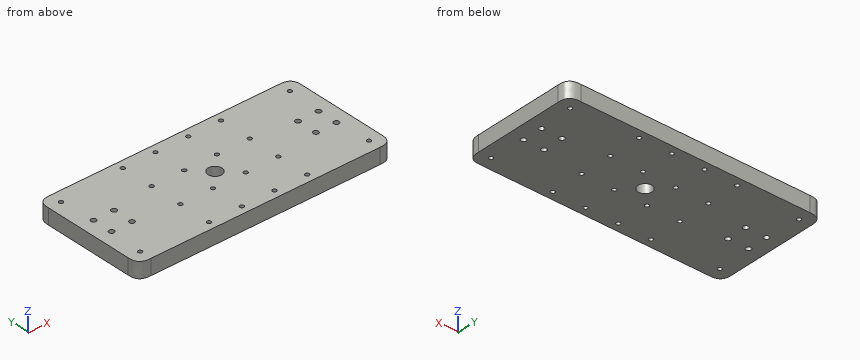
from build123d import *

# Parameters (mm, degrees)
SKETCH1_W                           = 310
SKETCH1_H                           = 140
BOSS_EXTRUDE1_DEPTH                 = 19.05
TAP_DRILL_FOR_M6X1_0_TAP1_D         = 5
LPATTERN1_COUNT                     = 4
LPATTERN1_PITCH                     = 40
LPATTERN1_COUNT_DIR2                = 4
LPATTERN1_PITCH_DIR2                = 40
FILLET1_SIZE                        = 15
M6_CLEARANCE_HOLE1_D                = 6.4
M16_CLEARANCE_HOLE1_D               = 17
TAP_START                           = -1
TAP_DRILL_FOR_M6X1_0_TAP2_OUTLINE_R = 2.5
TAP_DRILL_FOR_M6X1_0_TAP2_DEPTH     = 21


with BuildPart() as part:
    # Sketch1 → Boss-Extrude1 (new body)
    with BuildSketch(Plane.XY):
        Rectangle(SKETCH1_W, SKETCH1_H)
    extrude(amount=BOSS_EXTRUDE1_DEPTH)

    # Tap Drill for M6x1.0 Tap1 (through all)
    with Locations(Plane.XY.offset(19.05)):
        with Locations((-60, 60)):
            tap_drill_for_m6x1_0_tap1 = Hole(TAP_DRILL_FOR_M6X1_0_TAP1_D / 2)

    # LPattern1: Tap Drill for M6x1.0 Tap1 4 × 4
    with Locations(*[(i * LPATTERN1_PITCH, -j * LPATTERN1_PITCH_DIR2, 0) for i in range(LPATTERN1_COUNT) for j in range(LPATTERN1_COUNT_DIR2) if (i, j) != (0, 0)]):
        add(tap_drill_for_m6x1_0_tap1, mode=Mode.SUBTRACT)

    # Fillet1
    # a fillet whose section is not a circle: 15 mm, written as the material it takes off along each edge
    with BuildSketch(Plane(origin=(155, -70, -37.5), x_dir=(0, 1, 0), z_dir=(0, 0, 1)), Plane(origin=(155, 70, -37.5), x_dir=(-1, 0, 0), z_dir=(0, 0, 1))) as fillet1_piece_1:
        with BuildLine():
            add(Edge.make_bspline([(FILLET1_SIZE, 0), (FILLET1_SIZE * 0.831801948466, 0), (FILLET1_SIZE * 0.663603896932, 0), (FILLET1_SIZE * 0.292893218813, FILLET1_SIZE * 0.0716919198361), (FILLET1_SIZE * 0.0716919198361, FILLET1_SIZE * 0.292893218813), (0, FILLET1_SIZE * 0.663603896932), (0, FILLET1_SIZE * 0.831801948466), (0, FILLET1_SIZE)], knots=[0, 0, 0, 0, 0, 0, 0.5, 0.5, 1, 1, 1, 1, 1, 1], degree=5))
            Line((0, FILLET1_SIZE), (0, 0))
            Line((0, 0), (FILLET1_SIZE, 0))
        make_face()
    extrude(amount=94.05, mode=Mode.SUBTRACT)
    with BuildSketch(Plane(origin=(-155, 70, -37.5), x_dir=(1, 0, 0), z_dir=(0, 0, 1)), Plane(origin=(-155, -70, -37.5), x_dir=(0, 1, 0), z_dir=(0, 0, 1))) as fillet1_piece_2:
        with BuildLine():
            add(Edge.make_bspline([(FILLET1_SIZE, 0), (FILLET1_SIZE * 0.831801948466, 0), (FILLET1_SIZE * 0.663603896932, 0), (FILLET1_SIZE * 0.292893218813, -FILLET1_SIZE * 0.0716919198361), (FILLET1_SIZE * 0.0716919198361, -FILLET1_SIZE * 0.292893218813), (0, -FILLET1_SIZE * 0.663603896932), (0, -FILLET1_SIZE * 0.831801948466), (0, -FILLET1_SIZE)], knots=[0, 0, 0, 0, 0, 0, 0.5, 0.5, 1, 1, 1, 1, 1, 1], degree=5))
            Line((0, -FILLET1_SIZE), (0, 0))
            Line((0, 0), (FILLET1_SIZE, 0))
        make_face()
    extrude(amount=94.05, mode=Mode.SUBTRACT)

    # M6 Clearance Hole1 (through all)
    with Locations(Plane(origin=(0, 0, 0), x_dir=(-1, 0, 0), z_dir=(0, 0, -1))):
        with Locations((137.5, -12.5), (137.5, 12.5), (112.5, 12.5), (112.5, -12.5), (-112.5, -12.5), (-137.5, -12.5), (-112.5, 12.5), (-137.5, 12.5)):
            Hole(M6_CLEARANCE_HOLE1_D / 2)

    # M16 Clearance Hole1 (through all)
    with Locations(Plane.XY.offset(19.05)):
        with Locations((0, 0)):
            Hole(M16_CLEARANCE_HOLE1_D / 2)

    # Tap Drill for M6x1.0 Tap2: read off the stored shape, not the designer's step
    # Tap Drill for M6x1.0 Tap2 outline → Tap Drill for M6x1.0 Tap2 (cut)
    with BuildSketch(Plane.XY.offset(TAP_START)):
        with Locations((140, 55)):
            Circle(TAP_DRILL_FOR_M6X1_0_TAP2_OUTLINE_R)
        with Locations((-140, -55)):
            Circle(TAP_DRILL_FOR_M6X1_0_TAP2_OUTLINE_R)
        with Locations((140, -55)):
            Circle(TAP_DRILL_FOR_M6X1_0_TAP2_OUTLINE_R)
        with Locations((-140, 55)):
            Circle(TAP_DRILL_FOR_M6X1_0_TAP2_OUTLINE_R)
    extrude(amount=TAP_DRILL_FOR_M6X1_0_TAP2_DEPTH, mode=Mode.SUBTRACT)


solid = part.part
CAD build for the part. Positions are in the model's coordinates, mm. Round coordinates to 2 decimals unless told otherwise and drop trailing zeros. Write each loop counter-clockwise with the first axis right and the second up, starting at its lowest first coordinate (ties: lowest second). Pieces come first, ordered by that corner, then holes. Notation, with made-up numbers: M 53,-32 L 69,-32 A7 ccw 69,-25 Z; hole C -23,66 d3. An arc over 180 degrees is marked long. Put each result on its own line as item: value. Start each with the question number.
1) Saw through at D-D, the plane z = 8. Count the separate pieces of the cut face and the enclosed holes in it, and give its area (3 significant figures).
2) Pin check, flat tip, straight feed: pin 1 Ø4 at (x, y) = (-15, 36.5) entering from -Z. Stop position of the tip, or through.
3) Saw through at A-A, the plane y = 12.5. Write the cut outline in (x, z).
4) Saw through at B-B, the plane x = 0. Write the cut outline in (y, z).
5) Saw through at C-C, the plane x = 112.5. Write the cut outline in (y, z), and give its area (3 significant figures).
6) Drill centre lines: probe 1 along Y at (x, z) = (-60, 8.5); probe 2 along Y at (x, z) = (112.5, 5); probe 3 along Y at (x, z) = (-141, 8.75). Where is each one in solid material? Low to high. Write a range as [from, to].
Resolved:
1. separate pieces: 1
1. enclosed holes: 29
1. area: 42,400 mm²
2. pin 1: z = 0
3. outline: M -155,0 L -140.7,0 L -140.7,19.05 L -155,19.05 Z; M -134.3,0 L -115.7,0 L -115.7,19.05 L -134.3,19.05 Z; M -109.3,0 L 109.3,0 L 109.3,19.05 L -109.3,19.05 Z; M 115.7,0 L 134.3,0 L 134.3,19.05 L 115.7,19.05 Z; M 140.7,0 L 155,0 L 155,19.05 L 140.7,19.05 Z
4. outline: M -70,0 L -8.5,0 L -8.5,19.05 L -70,19.05 Z; M 8.5,0 L 70,0 L 70,19.05 L 8.5,19.05 Z
5. outline: M -70,0 L -15.7,0 L -15.7,19.05 L -70,19.05 Z; M -9.3,0 L 9.3,0 L 9.3,19.05 L -9.3,19.05 Z; M 15.7,0 L 70,0 L 70,19.05 L 15.7,19.05 Z
5. area: 2,420 mm²
6. probe 1: [-70, -62.5], [-57.5, -22.5], [-17.5, 17.5], [22.5, 57.5], [62.5, 70]
6. probe 2: [-70, -15.7], [-9.3, 9.3], [15.7, 70]
6. probe 3: [-70, -57.29], [-52.71, 52.71], [57.29, 70]
